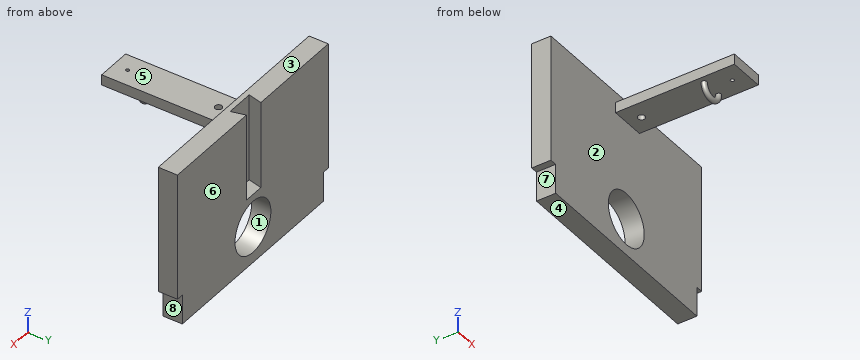
```python
from build123d import *

# Parameters (mm, degrees)
F0_R      = 7.5
F1_DEPTH  = 5.5
F3_DEPTH  = 25
F4_W      = 10
F4_H      = 3
F5_DEPTH  = 34
F6_R      = 0.5
F7_DEPTH  = 6
F6_R_2    = 1
F8_DEPTH  = 25
F9_R      = 0.75
F10_ANGLE = 180


# Not quite as in the source:
# - a feature names something its author has since deleted; it is built from what else it names


with BuildPart() as f1:
    # F0 (on Front) → F1 (new body)
    with BuildSketch(Plane.XZ):
        Polygon((0, 8.5), (0, 0), (59, 0), (59, 8.5), (61, 8.5), (61, 45), (-2, 45), (-2, 8.5), align=None)
        with Locations((29.5, 10.5)):
            Circle(F0_R, mode=Mode.SUBTRACT)
    extrude(amount=F1_DEPTH)

    # F2 (on face) → F3 (cut)
    with BuildSketch(Plane.XY.offset(45)):
        Polygon((26.2, 0), (25.2, -4), (33.2, -4), (32.2, 0), align=None)
    extrude(amount=-F3_DEPTH, mode=Mode.SUBTRACT)

    # F4 (on face) → F5 (join)
    with BuildSketch(Plane.XZ.offset(5.5)):
        with Locations((30, 40.5)):
            Rectangle(F4_W, F4_H)
    extrude(amount=F5_DEPTH)

    # F6 (on face) → F7 (cut)
    with BuildSketch(Plane.XY.offset(42)):
        with Locations((30, -35.5)):
            Circle(F6_R)
    extrude(amount=-F7_DEPTH, mode=Mode.SUBTRACT)

    # F6 (on face) → F8 (cut)
    with BuildSketch(Plane.XY.offset(42)):
        with Locations((30, -9.5)):
            Circle(F6_R_2)
    extrude(amount=-F8_DEPTH, mode=Mode.SUBTRACT)

    # F9 (on face) → F10 (revolve)
    with BuildSketch(Plane(origin=(0, 0, 39), x_dir=(1, 0, 0), z_dir=(0, 0, -1))):
        with Locations((33, 29.5)):
            Circle(F9_R)
    revolve(axis=Axis((30, -12.9445128906, 39), (0, 1, 0)), revolution_arc=F10_ANGLE)


solid = f1.part
```
CAD build for the part. Positions are in the model's coordinates, mm. Face numbers are marked on the shaded views. A direction names the side the tool comes from. Round coordinates to 2 decimals unless told otherwise and drop trailing zeros. Write each loop counter-clockwise with the first axis right and the second up, starting at its lowest first coordinate (ties: lowest second). Pieces come first, ordered by that corner, then holes. Notation, with made-up numbers: (23, -36) - (47, -36) arc R25 ccw to (47, -12) - close; hole circle Ø8 at (-20.5, 51.25). An arc over 180 degrees is marked (long way). Return JSON: item names as keys, results as strings. Group by question number.
Item 1: Band-saw the part on B-B on z = 22. List the corners of the cut face in (x, y), plus the area to 4 significant figures.
Item 2: Probe probe 1 along Y at (x, z) = (30, 40); probe 2 along X at (y, z) = (-35.5, 41.15); probe 3 along Y at (x, z) = (50, 30). List the from-to ranges inside material, lowest first.
Item 3: Flat gauge pins, fed straight in: pin 1 Ø2.5 at (y, z) = (-30.5, 40) entering from +X; pin 2 Ø5 at (x, y) = (31, -17.5) entering from -Z; pin 3 Ø10 at (x, z) = (20.5, 11.5) entering from -Y; pin 4 Ø12 at (x, z) = (29.5, 10.5) entering from -Y. Where does each tip first touch, or does it go through?
Item 4: Band-saw the part on A-A on y = -9.5. List the corners of the cut face in (x, z), plus the area to 3 significant figures.
Item 5: Band-saw the part on C-C on z = 13. List the corners of the cut face in (x, y).
Item 6: Mould opens along Z. For the marked faces 1, 2, 3 and 4 say: +Z half, -Z half, draft (parallel to the pull), parting line (faces both ways), or undercut.
Item 7: Band-saw the part on D-D on x = 40.5. List the corners of the cut face in (y, z), plus the area to 4 significant figures.
Item 8: 3-axis set-ups, long thin cutter, end or side, ignore diameter. For the marked faces 5, 6, 7 and 8: which of +Z, -Z, +X, -X, +Y, -Y reach the whole face in a straight line?
Resolved:
{
 "1": {"outline": "(-2, -5.5) - (61, -5.5) - (61, 0) - (32.2, 0) - (33.2, -4) - (25.2, -4) - (26.2, 0) - (-2, 0) - close", "area": "318.5 mm²"},
 "2": {"probe 1": "y = -39.5 to -36, -35 to -10.5, -8.5 to -4", "probe 2": "x = 25 to 29.5, 30.5 to 35", "probe 3": "y = -5.5 to 0"},
 "3": {"pin 1": "stops at x = 35", "pin 2": "stops at z = 39", "pin 3": "stops at y = -5.5", "pin 4": "passes through"},
 "4": {"outline": "(25, 39) - (29, 39) - (29, 42) - (25, 42) - close; (31, 39) - (35, 39) - (35, 42) - (31, 42) - close", "area": "24.0 mm²"},
 "5": {"outline": "(-2, -5.5) - (22.43, -5.5) - (22.43, 0) - (-2, 0) - close; (36.57, -5.5) - (61, -5.5) - (61, 0) - (36.57, 0) - close"},
 "6": {"face 1": "undercut", "face 2": "draft", "face 3": "+Z half", "face 4": "-Z half"},
 "7": {"outline": "(-5.5, 0) - (0, 0) - (0, 45) - (-5.5, 45) - close", "area": "247.5 mm²"},
 "8": {"face 5": "+Z, +X, -X, -Y", "face 6": "+Z, -Z, +X, -X, +Y", "face 7": "-Z, -X, +Y, -Y", "face 8": "-Z, +X, +Y, -Y"}
}
